Could you check a few things on this model? Use its own coordinates, in mm. A direction names the side the tool comes from. Coordinates: 2 decimals unless noted, no trailing zeros. Loops run counter-clockwise (first coordinate to the right, second up) from the corner with the lowest first, then second, coordinate; pieces in that order, holes last. Notation, with made-up numbers: (-8, -26.75) - (20, -26.75) arc R26 cw to (20, 3.25) - close; hole circle Ø2 at (-6, 45.5). An arc over 180 degrees is marked (long way). One line per question, with ' | ' between items. Start each with the question number.
1. Please list where these lines run through material, in increasing order: L1, parallel to X at y = 13, z = 0; L2, parallel to Y at x = 0, z = -2.1; L3, parallel to Z at x = 0, y = 9.25. Write a range as [from, to].
2. We'd pull the mould along Z, two halves only. Please class faces 1 (the flat face through (-2.96, 14.84, 5.22)), 2 (the cylindrical face through (0, 13, 2)), 3 (the flat face through (-3.042, 14.843, -5.172)): pulls with the +Z half, pulls with the -Z half, needs draft (parallel to the pull), parting line crosses it, or undercut.
3. Which directions (+Z, -Z, +X, -X, +Y, -Y) give clear straight access to the entire face, cutting with the end or side of a thin tool? Please do faces 4 (the cylindrical face through (-2, 5.45, -3.47)), 5 (the cylindrical face through (-5.484, 6.068, -1.727)).
4. I'm going to push flat-ended pins straight in: P1, Ø2.5, axis at x = 0, y = 5.37, coming from the +Z side; P2, Ø6.5, axis at x = 0, y = 5.37, coming from the -Z side; P3, Ø1.5, axis at x = 1, y = 6.5, coming from the +Z side; P4, Ø1.5, axis at y = 12, z = 5.5, coming from the -X side. Where does each tip first touch, or does it pass through?
5. I want a section at A-A, the plane y = 12.5. Write out the boundary of the cut face in (x, z), then the cut area to 3 significant figures.
Autodesk Inventor part; units mm, degrees
ref_plane "YZ Plane" through (0, 0, 0) normal (1, 0, 0) x (0, 1, 0)
ref_plane "XZ Plane" through (0, 0, 0) normal (0, 1, 0) x (-1, 0, 0)
ref_plane "XY Plane" through (0, 0, 0) normal (0, 0, 1) x (1, 0, 0)
sketch "Sketch1" plane through (0, 0, 0) normal (0, 1, 0) x (-1, 0, 0)
  circle A0 centre (0, 0) radius 5.75
  circle A1 centre (0, 0) radius 2
  dimension "d0" = 4
  dimension "d1" = 11.5
extrude "Extrusion1" add sketch "Sketch1" along normal blind 12
sketch "Sketch2" plane through (0, 12, 0) normal (0, 1, 0) x (1, 0, 0)
  circle A0 centre (0, 0) radius 2
  line L0 (0, 6.9282) -> (6, 3.4641)
  line L1 (6, 3.4641) -> (6, -3.4641)
  line L2 (6, -3.4641) -> (0, -6.9282)
  line L3 (0, -6.9282) -> (-6, -3.4641)
  line L4 (-6, -3.4641) -> (-6, 3.4641)
  line L5 (-6, 3.4641) -> (0, 6.9282)
  dimension "d4" = 12
extrude "Extrusion2" add sketch "Sketch2" along normal blind 6
chamfer "Chamfer1" distance 0.3 angle 45 1 edges at (5.75, 0, 0)
sketch "Sketch3" plane through (0, 0, 0) normal (1, 0, 0) x (0, 1, 0)
  line L0 (16.8879, 9.0352) -> (19.8879, 9.0352)
  line L1 (18, 2) -> (18, -2)
  line L2 (18, 3.4641) -> (18, 6.9282)
  line L3 (-31.6303, 0) -> (26.5625, 0)
  line L4 (19.8879, 9.0352) -> (19.8879, 0)
  line L5 (19.8879, 0) -> (18, 0)
  arc A0 (18, 0) -> (16.8879, 9.0352) centre (-0.7575, 2.2772) ccw
  point P0 (0, 0)
  dimension "d10" = 9.0352
  dimension "d11" = 3
revolve "Revolution1" cut sketch "Sketch3" angle 360 about axis through (0, 0, 0) along (0, 1, 0)
sketch "Sketch4" plane through (0, 0, 0) normal (0, 0, 1) x (1, 0, 0)
  line L0 (0, 0) -> (0, 5.3666) construction
  circle A0 centre (0, 5.3666) radius 2
  dimension "d13" = 4
extrude "Extrusion3" cut sketch "Sketch4" against normal mid plane 30
thread "Thread1"
thread "Thread2"
properties part number "Coupler"
Results are:
1) L1: x = [-6, -2], [2, 6] | L2: y = [0, 3.37], [7.37, 18] | L3: z = [-5.75, -2], [2, 5.75]
2) face 1: pulls with the +Z half | face 2: undercut | face 3: pulls with the -Z half
3) face 4: +Z, -Z | face 5: -Y
4) P1: passes through | P2: stops at z = -5.75 | P3: stops at z = 5.7 | P4: stops at x = -3.77
5) outline: (-6, -3.46) - (0, -6.93) - (6, -3.46) - (6, 3.46) - (0, 6.93) - (-6, 3.46) - close; hole circle Ø4 at (0, 0) | area: 112 mm2
